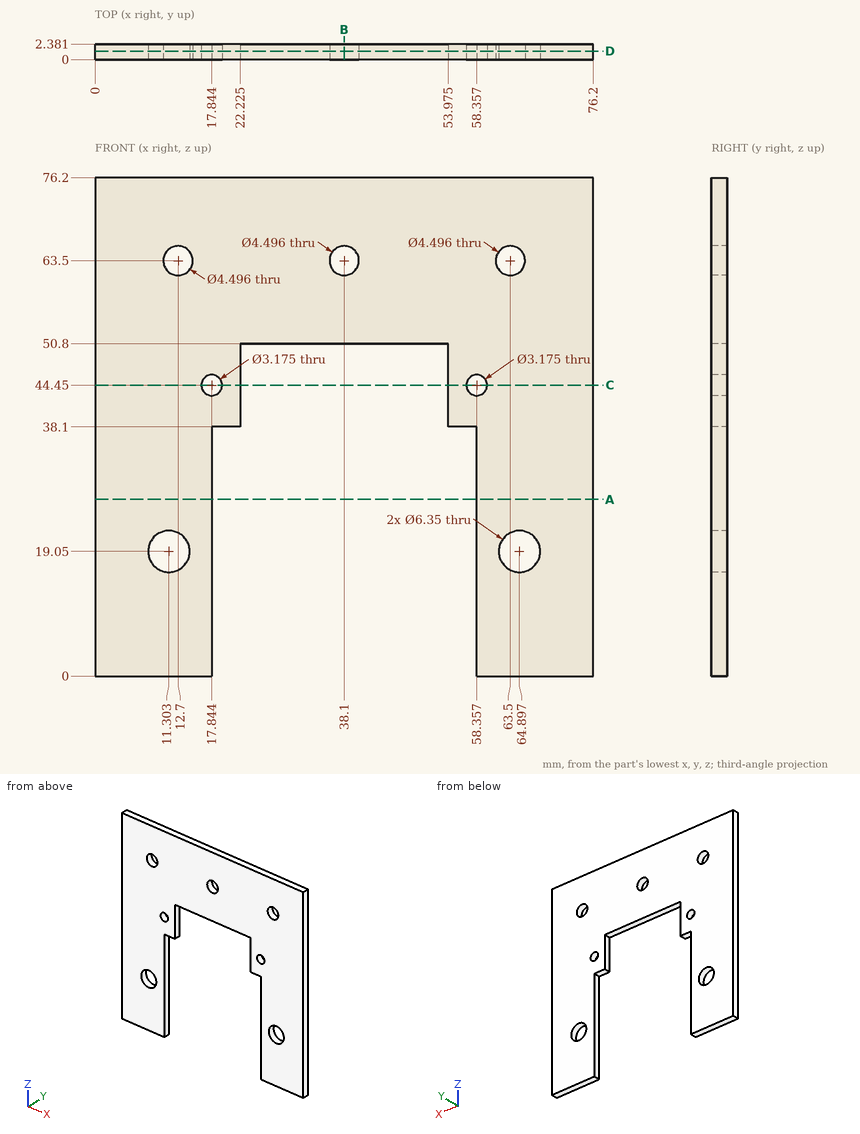
Source: three-view drawing plus pictorial views. Frame: mm from the lowest corner of the part. Round coordinates to 2 decimals unless told otherwise and drop trailing zeros. Loops run counter-clockwise (first coordinate to the right, second up) from the corner with the lowest first, then second, coordinate; pieces in that order, holes last. Notation, with made-up numbers: M 34.25,43 L 77.25,43 A33 cw 77.25,78 Z; hole C 38,89.25 d6. An arc over 180 degrees is marked long. Answer as CSV lines item,"result". Start each with the question number.
(1) First-contact query: pin 1 (1.2 mm diameter, centred on x = 34.5, y = 1.5, fed in from -Z); pin 2 (0.7 mm diameter, centred on x = 56.5, y = 1.5, fed in from -Z). Flat tips, straight axial feed; report the tip coordinate or a pass-through.
(2) Section B-B, the plane x = 38.1. Output: boundary loops of the cut face in (y, z).
(3) Section D-D, the plane y = 1.3. State how many separate pieces and enclosed holes the cut face has, plus the area to 3 significant figures.
(4) Line query: line 1 (X direction, y = 1.4, z = 44.45) (1 decimal); line 2 (X direction, y = 1.45, z = 63.5); line 3 (X direction, y = 1, z = 15). Output: solid intervals per line, ascending. Write a range as [from, to].
(5) Section C-C, the plane z = 44.45. Output: boundary loops of the cut face in (x, y) (1 decimal).
(6) Section A-A, the plane z = 27. Output: boundary loops of the cut face in (x, y).
Values found:
1,pin 1,"stops at z = 50.8"
1,pin 2,"stops at z = 38.1"
2,outline,"M 0,50.8 L 2.38,50.8 L 2.38,61.25 L 0,61.25 Z; M 0,65.75 L 2.38,65.75 L 2.38,76.2 L 0,76.2 Z"
3,separate pieces,"1"
3,enclosed holes,"7"
3,area,"3,730 mm²"
4,line 1,"x = [0, 16.3], [19.4, 22.2], [54, 56.8], [59.9, 76.2]"
4,line 2,"x = [0, 10.45], [14.95, 35.85], [40.35, 61.25], [65.75, 76.2]"
4,line 3,"x = [0, 17.84], [58.36, 76.2]"
5,outline,"M 0,0 L 16.3,0 L 16.3,2.4 L 0,2.4 Z; M 19.4,0 L 22.2,0 L 22.2,2.4 L 19.4,2.4 Z; M 54,0 L 56.8,0 L 56.8,2.4 L 54,2.4 Z; M 59.9,0 L 76.2,0 L 76.2,2.4 L 59.9,2.4 Z"
6,outline,"M 0,0 L 17.84,0 L 17.84,2.38 L 0,2.38 Z; M 58.36,0 L 76.2,0 L 76.2,2.38 L 58.36,2.38 Z"
